The listing builds one solid part. Answer for the finished solid, in the listing's coordinates (mm). Round coordinates to 2 decimals unless told otherwise and drop trailing zeros. Order: outer loops, then holes, each group sorted by start corner. A loop starts at its lowest first (then second) coordinate and runs counter-clockwise, first axis right, second up. Notation, with made-up numbers: (-8, 53.5) -> (46, 53.5) arc R20 cw to (46, 80.5) -> close; hole circle Ø6 at (17.5, 70.5). An arc over 180 degrees is marked (long way). Answer in a Markdown table with one row per item. Add a question column.
```python
from build123d import *

# Parameters (mm, degrees)
BOSS_EXTRUDE1_START           = 0.3
SKETCH1_W                     = 5
SKETCH1_H                     = 6
BOSS_EXTRUDE1_DEPTH           = 0.3
BOSS_EXTRUDE1_OTHER_WAY_DEPTH = 0.7
BOSS_EXTRUDE1_OTHER_WAY_TAPER = 11
FILLET1_R                     = 0.2
BOSS_EXTRUDE2_DEPTH           = 0.05
BOSS_EXTRUDE2_DEPTH_BACK      = 0.3
SKETCH3_W                     = 0.4
SKETCH3_H                     = 0.6


with BuildPart() as part:
    # Sketch1 → Boss-Extrude1 (new body)
    with BuildSketch(Plane.XY.offset(BOSS_EXTRUDE1_START)):
        Rectangle(SKETCH1_W, SKETCH1_H)
    extrude(amount=-BOSS_EXTRUDE1_DEPTH)

    # Sketch1 → Boss-Extrude1 other way (add)
    with BuildSketch(Plane.XY.offset(BOSS_EXTRUDE1_START)):
        Rectangle(SKETCH1_W, SKETCH1_H)
    extrude(amount=BOSS_EXTRUDE1_OTHER_WAY_DEPTH, taper=BOSS_EXTRUDE1_OTHER_WAY_TAPER)

    # Fillet1
    fillet1_edges = [part.edges().sort_by_distance(p)[0] for p in [
        (-2.363933784, 0, 1),
        (0, -2.863933784, 1),
        (2.363933784, 0, 1),
        (0, 2.863933784, 1),
    ]]
    fillet(fillet1_edges, radius=FILLET1_R)

    # Sketch3 → Boss-Extrude2 (add, two sides: drawn at the far end of the back side and taken through both)
    with BuildSketch(Plane(origin=(0, 0, 0), x_dir=(-1, 0, 0), z_dir=(0, 0, -1)).offset(-BOSS_EXTRUDE2_DEPTH_BACK)):
        with Locations((1.905, -2.825)):
            Rectangle(SKETCH3_W, SKETCH3_H)
        with Locations((0.635, -2.825)):
            Rectangle(SKETCH3_W, SKETCH3_H)
        with Locations((-0.635, -2.825)):
            Rectangle(SKETCH3_W, SKETCH3_H)
        with Locations((-1.905, -2.825)):
            Rectangle(SKETCH3_W, SKETCH3_H)
        Polygon((2.105, 2.525), (2.105, 3.125), (1.705, 3.125), (1.705, 2.525), (0.835, 2.525), (0.835, 3.125), (0.435, 3.125), (0.435, 2.525), (-0.435, 2.525), (-0.435, 3.125), (-0.835, 3.125), (-0.835, 2.525), (-1.705, 2.525), (-1.705, 3.125), (-2.105, 3.125), (-2.105, 2.525), (-2.2, 2.525), (-2.2, -0.775), (-2.6, -0.775), (-2.6, -1.075), (2.6, -1.075), (2.6, -0.775), (2.2, -0.775), (2.2, 2.525), align=None)
    extrude(amount=BOSS_EXTRUDE2_DEPTH + BOSS_EXTRUDE2_DEPTH_BACK)


solid = part.part
```
1. The part is cut by section B-B (x = 1.8). Give the vertices of the cut face in (y, z) (3 decimals).
2. Straight lines are drawn through the part: line 1 along Y through (x, z) = (-2.3, 0.2); line 2 along Z through (x, y) = (-0.6, -1.25); line 3 along X through (y, z) = (0.5, 0.1). For each, find the intervals that lie inside material, in ascending order.
3. The part is cut by section A-A (y = -2.25). Give the vertices of the cut face in (x, z).
4. The mould has two halves that part along Y. Classify faces 1 (the flat face through (0, 0, 1)), 2 (the flat face through (0, -2, 0)): released by +Y, released by -Y, zero draft, split by the parting line, or undercut.
5. The part is cut by section C-C (x = 1.1). Give the vertices of the cut face in (y, z) (3 decimals), then the cut area to 3 significant figures.
6. The part is cut by section D-D (z = 0.7). Give the vertices of the cut face in (x, y), then the cut area to 3 significant figures.
Report:
| question | item | result |
|---|---|---|
| 1 | outline | (-3.125, -0.05) -> (-2.525, -0.05) -> (-2.525, 0) -> (-1.075, 0) -> (-1.075, -0.05) -> (3.125, -0.05) -> (3.125, 0.3) -> (3, 0.3) -> (2.895, 0.838) arc R0.2 ccw to (2.699, 1) -> (-2.699, 1) arc R0.2 ccw to (-2.895, 0.838) -> (-3, 0.3) -> (-3.125, 0.3) -> close |
| 2 | line 1 | y = -3 to 3 |
| 2 | line 2 | z = 0 to 1 |
| 2 | line 3 | x = -2.5 to 2.5 |
| 3 | outline | (-2.5, 0) -> (2.5, 0) -> (2.5, 0.3) -> (2.4, 0.84) arc R0.2 ccw to (2.2, 1) -> (-2.2, 1) arc R0.2 ccw to (-2.4, 0.84) -> (-2.5, 0.3) -> close |
| 4 | face 1 | zero draft |
| 4 | face 2 | undercut |
| 5 | outline | (-3, 0) -> (-1.075, 0) -> (-1.075, -0.05) -> (2.525, -0.05) -> (2.525, 0) -> (3, 0) -> (3, 0.3) -> (2.895, 0.838) arc R0.2 ccw to (2.699, 1) -> (-2.699, 1) arc R0.2 ccw to (-2.895, 0.838) -> (-3, 0.3) -> close |
| 5 | area | 6.07 mm^2 |
| 6 | outline | (-2.42, -2.92) -> (2.42, -2.92) -> (2.42, 2.92) -> (-2.42, 2.92) -> close |
| 6 | area | 28.3 mm^2 |
